from build123d import *

# Parameters (mm, degrees)
BOSS_EXTRUDE1_DEPTH = 10
CUT_EXTRUDE1_DEPTH  = 3.8
SKETCH6_R           = 2.3
BOSS_EXTRUDE2_DEPTH = 1
SKETCH7_R           = 1.05
CUT_EXTRUDE2_DEPTH  = 57.699667466
SKETCH8_R           = 0.6
BOSS_EXTRUDE3_DEPTH = 3
SKETCH9_R           = 2
CUT_EXTRUDE4_DEPTH  = 6
SKETCH10_R          = 3.99955369
CUT_EXTRUDE7_DEPTH  = 3
CUT_EXTRUDE8_DEPTH  = 58.122782589
SKETCH15_R          = 5
BOSS_EXTRUDE4_DEPTH = 10


# Read off the part's stored shape, not the designer's step: Boss-Extrude1
with BuildPart() as part:
    # Boss-Extrude1 outline → Boss-Extrude1 (new body)
    with BuildSketch(Plane(origin=(0, 0, 0), x_dir=(1, 0, 0), z_dir=(0, 1, 0))):
        with BuildLine():
            Line((5, -55.344368806), (5, -50))
            Line((5, -50), (10, 0))
            ThreePointArc((10, 0), (0, 10), (-10, 0))
            Line((-10, 0), (-5, -50))
            Line((-5, -50), (-10.000656588, -52.844368806))
            Line((-10.000656588, -52.844368806), (-10.000656588, -55.344368806))
            Line((-10.000656588, -55.344368806), (5, -55.344368806))
        make_face()
    extrude(amount=BOSS_EXTRUDE1_DEPTH)

    # Sketch5 → Cut-Extrude1 (cut)
    with BuildSketch(Plane(origin=(0, 10, 0), x_dir=(1, 0, 0), z_dir=(0, 1, 0))):
        with BuildLine():
            Line((2, -14.05), (2.649226302, -2.21))
            ThreePointArc((2.649226302, -2.21), (0, 3.45), (-2.649226302, -2.21))
            Line((-2.649226302, -2.21), (-2, -14.05))
            ThreePointArc((-2, -14.05), (0, -16.05), (2, -14.05))
        make_face()
    extrude(amount=-CUT_EXTRUDE1_DEPTH, mode=Mode.SUBTRACT)

    # Sketch6 → Boss-Extrude2 (add)
    with BuildSketch(Plane(origin=(0, 6.2, 0), x_dir=(1, 0, 0), z_dir=(0, 1, 0))):
        with Locations(Location((0, 0, 0), (0, 0, 270))):
            Circle(SKETCH6_R)
    extrude(amount=BOSS_EXTRUDE2_DEPTH)

    # Sketch7 → Cut-Extrude2 (cut, through all)
    with BuildSketch(Plane(origin=(0, 7.2, 0), x_dir=(1, 0, 0), z_dir=(0, 1, 0))):
        with Locations(Location((0, 0, 0), (0, 0, 270))):
            Circle(SKETCH7_R)
    extrude(amount=-CUT_EXTRUDE2_DEPTH, mode=Mode.SUBTRACT)

    # Sketch8 → Boss-Extrude3 (add)
    with BuildSketch(Plane(origin=(0, 6.2, 0), x_dir=(1, 0, 0), z_dir=(0, 1, 0))):
        with Locations(Location((0, -4.45, 0), (0, 0, 270))):
            Circle(SKETCH8_R)
        with Locations(Location((0, -6.45, 0), (0, 0, 270))):
            Circle(SKETCH8_R)
        with Locations(Location((0, -8.45, 0), (0, 0, 270))):
            Circle(SKETCH8_R)
        with Locations(Location((0, -10.45, 0), (0, 0, 270))):
            Circle(SKETCH8_R)
        with Locations(Location((0, -12.45, 0), (0, 0, 270))):
            Circle(SKETCH8_R)
        with Locations(Location((0, -14.45, 0), (0, 0, 270))):
            Circle(SKETCH8_R)
    extrude(amount=BOSS_EXTRUDE3_DEPTH)

    # Sketch9 → Cut-Extrude4 (cut)
    with BuildSketch(Plane.XZ):
        with Locations(Location((0, 0, 0), (0, 0, 270))):
            Circle(SKETCH9_R)
    extrude(amount=-CUT_EXTRUDE4_DEPTH, mode=Mode.SUBTRACT)

    # Sketch10 → Cut-Extrude7 (cut)
    with BuildSketch(Plane(origin=(0, 10, 0), x_dir=(1, 0, 0), z_dir=(0, 1, 0))):
        Circle(SKETCH10_R)
    extrude(amount=-CUT_EXTRUDE7_DEPTH, mode=Mode.SUBTRACT)

    # Sketch14 → Cut-Extrude8 (cut, through all)
    with BuildSketch(Plane(origin=(0, 10, 0), x_dir=(1, 0, 0), z_dir=(0, 1, 0))):
        Polygon((-5, -50), (5, -50), (5, -55.344368806), (-10.000656588, -55.344368806), (-10.000656588, -52.844368806), align=None)
    extrude(amount=-CUT_EXTRUDE8_DEPTH, mode=Mode.SUBTRACT)

    # Sketch15 → Boss-Extrude4 (add)
    with BuildSketch(Plane(origin=(0, 10, 0), x_dir=(1, 0, 0), z_dir=(0, 1, 0))):
        with Locations((0, -50)):
            Circle(SKETCH15_R)
    extrude(amount=-BOSS_EXTRUDE4_DEPTH)


solid = part.part
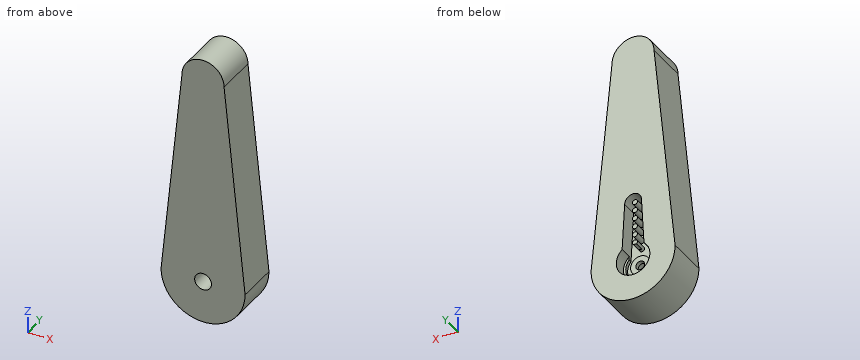
Build history of the part. All positions in model axes, mm. Coordinates: 2 decimals unless noted, no trailing zeros. Order: outer loops, then holes, each group sorted by start corner. A loop starts at its lowest first (then second) coordinate and runs counter-clockwise, first axis right, second up. Notation, with made-up numbers: (52, 28.5) - (62, 28.5) arc R10 ccw to (62, 37.5) - close; hole circle Ø1 at (-14.5, 18). An arc over 180 degrees is marked (long way). Write each question's results on one line, items separated by ' | '. Start each with the question number.
Item 1: Band-saw the part on A-A on y = 8. Write the cut outline in (x, z).
Item 2: Wall check: probe 1 along X at (y, z) = (6.75, 0); probe 2 along X at (y, z) = (8.9, 0); probe 3 along X at (y, z) = (2.25, 0). Give the ranges that are in metal, low to high. Write a range as [from, to].
Item 3: Band-saw the part on D-D on z = 18.5. Write the cut outline in (x, y).
Item 4: Band-saw the part on B-B on z = 10.45. Write the cut outline in (x, y) (3 decimals), and give its area (3 significant figures).
Item 5: Band-saw the part on C-C on y = 1.25. Write the cut outline in (x, z).
Item 6: Flat gauge pins, fed straight in: pin 1 (1.2 mm diameter, centred on x = 0, z = 4.5, fed in from +Y); pin 2 (5 mm diameter, centred on y = 4, z = 28, fed in from -X); pin 3 (4.5 mm diameter, centred on x = 0, z = 0, fed in from +Y). Where does each tip first touch, or does it go through?
Numbers:
1) outline: (-10, 0) arc R10 ccw to (10, 0) - (5, 50) arc R5 ccw to (-5, 50) - close; circle Ø1.2 at (0, 6.45); circle Ø1.2 at (0, 8.45); circle Ø1.2 at (0, 10.45); circle Ø1.2 at (0, 12.45); circle Ø1.2 at (0, 14.45); (-0.38, 3.98) arc R4 cw to (0.38, 3.98) arc R0.6 ccw (long way) to start; hole (-2.6, 3.04) arc R4 ccw (long way) to (2.6, 3.04) - (2, 14.05) arc R2 ccw to (-2, 14.05) - close
2) probe 1: [-10, -3.45], [-2.3, -1.05], [1.05, 2.3], [3.45, 10] | probe 2: [-10, -4], [4, 10] | probe 3: [-10, -2], [2, 10]
3) outline: (-8.15, 0) - (8.15, 0) - (8.15, 10) - (-8.15, 10) - close
4) outline: (-8.955, 0) - (8.955, 0) - (8.955, 10) - (2.197, 10) - (2.197, 6.2) - (0.6, 6.2) - (0.6, 9.2) - (-0.6, 9.2) - (-0.6, 6.2) - (-2.197, 6.2) - (-2.197, 10) - (-8.955, 10) - close | area: 166 mm^2
5) outline: (-10, 0) arc R10 ccw to (10, 0) - (5, 50) arc R5 ccw to (-5, 50) - close; hole circle Ø4 at (0, 0)
6) pin 1: y = 9.2 | pin 2: x = -7.45 | pin 3: y = 7
